Here's how the part is built. I have some questions about the finished solid (model axes, mm). A direction names the side the tool comes from. Coordinates: 2 decimals unless noted, no trailing zeros. Use a Markdown table: item, result.
Autodesk Inventor part; units mm, degrees
ref_plane "YZ Plane" through (0, 0, 0) normal (1, 0, 0) x (0, 1, 0)
ref_plane "XZ Plane" through (0, 0, 0) normal (0, 1, 0) x (-1, 0, 0)
ref_plane "XY Plane" through (0, 0, 0) normal (0, 0, 1) x (1, 0, 0)
sketch "Sketch1" plane through (0, 0, 0) normal (0, 1, 0) x (-1, 0, 0)
  arc A0 (5, 25) -> (25, 5) centre (25, 25) ccw
  circle A1 centre (25, 25) radius 20
  arc A2 (0, 10) -> (10, 0) centre (10, 10) ccw
  circle A3 centre (10, 10) radius 10
  line L0 (5.8856, 19.1144) -> (0, 19.1144)
  line L1 (0, 90) -> (0, 10)
  line L2 (19.1144, 5.8856) -> (19.1144, 0)
  line L3 (10, 0) -> (190, 0)
  line L4 (0, 19.1144) -> (19.1144, 19.1144)
  line L5 (19.1144, 19.1144) -> (19.1144, 0)
  line L6 (19.1144, 0) -> (0, 0)
  line L7 (0, 0) -> (0, 19.1144)
  arc A4 (45, 75) -> (5, 75) centre (25, 75) ccw
  circle A5 centre (25, 75) radius 20
  line L8 (25, 75) -> (25, 25)
  line L9 (25, 75) -> (35, 75)
  line L10 (35, 75) -> (35, 50)
  line L11 (35, 50) -> (25, 50)
  line L12 (25, 50) -> (25, 75)
  circle A6 centre (25, 75) radius 20
  line L13 (19.1144, 80.8856) -> (19.1144, 100)
  line L14 (0, 80.8856) -> (19.1144, 80.8856)
  line L15 (0, 100) -> (0, 80.8856)
  line L16 (19.1144, 100) -> (0, 100)
  circle A7 centre (10, 90) radius 10
  line L17 (19.1144, 0) -> (169.1144, 0) construction
  line L18 (-101.8121, -91.2055) -> (-91.2055, -101.8121)
  line L19 (0, 0) -> (-96.5088, -96.5088)
  line L20 (-96.5088, -96.5088) -> (-91.2055, -101.8121)
  line L21 (-91.2055, -101.8121) -> (-101.8121, -91.2055)
  line L22 (-91.2055, -101.8121) -> (10.6066, 0)
  line L23 (-101.8121, -91.2055) -> (0, 10.6066)
  line L24 (0, 19.1144) -> (-101.8121, -91.2055)
  line L25 (19.1144, 0) -> (-91.2055, -101.8121)
  point P0 (19.1144, 5.8856)
  point P1 (5.8856, 19.1144)
  point P2 (10, 100)
  point P3 (5.8856, 80.8856)
  point P4 (19.1144, 94.1144)
  point P5 (5.8856, 19.1144)
  point P6 (19.1144, 5.8856)
  dimension "d0" = 10
  dimension "d1" = 25
extrude "Extrusion1" add sketch "Sketch1" along normal blind 35 contours A0 A3 A2 | A3 L1 L0 | L2 L3 A3 | L7 L19 L18 L23 L1 | A2 L6 L7 | L1 L23 L24 | L3 L22 L18 L19 L6 | L25 L22 L3
sketch "Sketch3" plane through (0, 0, 0) normal (0, -1, 0) x (1, 0, 0)
  arc A0 (-19.1144, 5.8856) -> (-5.8856, 19.1144) centre (-25, 25) ccw
  circle A1 centre (-25, 25) radius 20
  line L0 (0, 0) -> (-19.1144, 0)
  line L1 (-19.1144, 0) -> (-19.1144, 19.1144)
  line L2 (-19.1144, 19.1144) -> (0, 19.1144)
  line L3 (0, 19.1144) -> (0, 0)
  line L4 (91.2055, -101.8121) -> (-19.1144, 0)
  line L5 (-5.8856, 19.1144) -> (0, 19.1144)
  line L6 (-19.1144, 0) -> (0, 19.1144)
  line L7 (-19.1144, 19.1144) -> (0, 0)
  point P0 (-5.8856, 19.1144)
  point P1 (-19.1144, 5.8856)
extrude "Extrusion4" cut sketch "Sketch3" against normal blind 20 contours A0 L7 L6 L1 | A0 L2 L6 L7 | L6 L7 L0 | L6 L3 L7
fillet "Fillet2" radius 10 1 edges at (0, 10, 0)
sketch "Sketch6" plane through (91.2055, 0, -101.8121) normal (-0.6782, 0, -0.7349) x (-0.7349, 0, 0.6782)
  line L0 (150.1206, 20) -> (150.1206, 35)
  line L1 (150.1206, 35) -> (136.6046, 35)
  line L2 (0, 35) -> (150.1206, 35)
  line L3 (143.4227, 0) -> (150.1206, 0)
  line L4 (0, 35) -> (150.1206, 35)
  line L5 (150.1206, 35) -> (150.1206, 0)
  line L6 (150.1206, 0) -> (0, 0)
  line L7 (0, 0) -> (0, 35)
  line L8 (0, 0) -> (150.1206, 0)
  line L9 (0, 0) -> (0, 10)
  line L10 (0, 0) -> (10, 0) construction
  line L11 (0, 10) -> (136.6046, 35)
  line L12 (0, 10) -> (-15.7766, 7.1127)
  line L13 (-15.7766, 7.1127) -> (-15.4206, 35)
  line L14 (0, 0) -> (0, 35)
  line L15 (-15.4206, 35) -> (0, 35)
  point P0 (136.0739, 0)
  dimension "d22" = 13.516
  dimension "d23" = 10
  dimension "d24" = 90
extrude "Extrusion5" cut sketch "Sketch6" against normal through all contours L11 L7 L2 | L7 L12 L13 L15
sketch "Sketch7" plane through (0, 20, 0) normal (0, -1, 0) x (1, 0, 0)
  line L0 (0, 0) -> (200, 0)
  line L1 (200, 0) -> (200, 100)
  line L2 (200, 100) -> (0, 100)
  line L3 (0, 100) -> (0, 0)
  line L4 (0, 0) -> (7, 0)
  line L5 (7, 0) -> (7, 7)
  line L6 (7, 7) -> (0, 7)
  line L7 (0, 7) -> (0, 0)
  line L8 (200, 100) -> (193, 100)
  line L9 (193, 100) -> (193, 93)
  line L10 (193, 93) -> (200, 93)
  line L11 (200, 93) -> (200, 100)
  line L12 (7, 7) -> (193, 7)
  line L13 (193, 7) -> (193, 93)
  line L14 (193, 93) -> (7, 93)
  line L15 (7, 93) -> (7, 7)
  line L16 (0, 0) -> (-200, 0)
  line L17 (-200, 0) -> (-200, 100)
  line L18 (-200, 100) -> (0, 100)
  line L19 (0, 0) -> (-7, 0)
  line L20 (-7, 0) -> (-7, 7)
  line L21 (-7, 7) -> (0, 7)
  line L22 (-200, 100) -> (-193, 100)
  line L23 (-193, 100) -> (-193, 93)
  line L24 (-193, 93) -> (-200, 93)
  line L25 (-200, 93) -> (-200, 100)
  line L26 (-7, 7) -> (-193, 7)
  line L27 (-193, 7) -> (-193, 93)
  line L28 (-193, 93) -> (-7, 93)
  line L29 (-7, 93) -> (-7, 7)
  dimension "d27" = 200
  dimension "d28" = 100
  dimension "d29" = 7
  dimension "d30" = 7
  dimension "d31" = 7
  dimension "d32" = 7
hole "Hole1" at (-7, 20, 7) direction (0, 1, 0) diameter 5 end through all
fillet "Fillet3" radius 5 1 edges at (96.5088, 9.945, -96.5088)
fillet "Fillet4" radius 5 4 edges at (90.3527, 9.0335, -101.025) (91.2055, 2.9156, -101.8121) (101.025, 8.9228, -90.3527) (101.8121, 2.8606, -91.2055)
sketch "Sketch8" plane through (0, 0, 0) normal (0, -1, 0) x (1, 0, 0)
  line L0 (98.4155, -94.6021) -> (94.6021, -98.4155)
  line L1 (98.4155, -94.6021) -> (103.9755, -89.0422)
  line L2 (0, 19.1144) -> (98.5544, -87.6756)
  line L3 (98.5544, -87.6756) -> (108.5515, -97.6726)
  ellipse E0 centre (94.88, -91.0666) end of major axis (91.3445, -87.531) minor radius 0.0367 (98.4155, -94.6021) -> (95.5415, -91.677) ccw
  line L4 (98.4155, -94.6021) -> (90.1473, -102.8703)
  line L5 (87.6756, -98.5544) -> (-19.1144, 0)
  line L6 (87.6756, -98.5544) -> (92.1576, -103.0365)
  circle A0 centre (90.9886, -90.9886) radius 7.8068
  circle A1 centre (90.9886, -90.9886) radius 20
  point P0 (0, 0)
  point P1 (98.0828, -94.2471)
  point P2 (96.5088, -96.5088)
  dimension "d42" = 40
extrude "Extrusion6" add sketch "Sketch8" against normal blind 5 contours L1 L3 L2 A1 L5 L6 L4 L0 | E0 A0 L2 L3 L1 | L0 L4 L6 L5 A0 | A0 | L5 A1 L2 A0
fillet "Fillet5" radius 5 1 edges at (105.1307, 5, -105.1307)
sketch "Sketch9" plane through (0, 0, 0) normal (0, -1, 0) x (1, 0, 0)
  arc A0 (72.1624, -84.2376) -> (84.2376, -72.1624) centre (90.9886, -90.9886) ccw
  circle A1 centre (90.9886, -90.9886) radius 4.25
  point P0 (0, 0)
  dimension "d46" = 8.5
extrude "Extrusion7" cut sketch "Sketch9" against normal through all
sketch "Sketch10" plane through (0, 0, 0) normal (0, -1, 0) x (1, 0, 0)
  circle A0 centre (90.9886, -90.9886) radius 4.25
  circle A1 centre (90.9886, -90.9886) radius 4.25
  circle A2 centre (90.9886, -90.9886) radius 2.5
  point P0 (0, 0)
  dimension "d49" = 5
extrude "Extrusion8" add sketch "Sketch10" against normal blind 5
properties part number "Noga"
Q1. If we mould it in two halves opening along Z, with no side actions, what happens to faces 4 (the face through (-4, 35, 7)), 5 (the face through (93, 5, -93)), 6 (the face through (-10.955, 27.395, 10.762))? For each: pulls with the +Z half, pulls with the -Z half, needs draft (parallel to the pull), parting line crosses it, or undercut.
Check values:
| item | result |
|---|---|
| face 4 | needs draft |
| face 5 | undercut |
| face 6 | pulls with the +Z half |
Q2. Which directions (+Z, -Z, +X, -X, +Y, -Y) give clear straight access to the entire face, cutting with the end or side of a thin tool? Please do faces 1 (the face through (97, 5, -97)), 2 (the face through (0, 10, 15)), 3 (the face through (35.091, 25.855, -34.872)).
Check values:
| item | result |
|---|---|
| face 1 | +Y |
| face 2 | +Z, -X, -Y |
| face 3 | -Z, +X, +Y |
Q3. Will these pins go through, and if not, where does the flat tip stop? P1, Ø4, axis at x = 91.5, z = -89.5, coming from the +Y side; P2, Ø4.5, axis at y = 8.5, z = 13, coming from the -X side; P3, Ø6, axis at y = 14, z = -74.5, coming from the +X side; P4, Ø8, axis at y = 28.5, z = -51.5, coming from the -X side.
Check values:
| item | result |
|---|---|
| P1 | y = 5 |
| P2 | x = 0 |
| P3 | x = 86.87 |
| P4 | through |
Q4. Please list where these lines run through material, in increasing order: L1, parallel to Y at x = 93, z = -102; L2, parallel to Y at x = 37, z = -22; L3, parallel to X at y = 20, z = -3. Write a range as from..to.
Check values:
| item | result |
|---|---|
| L1 | 0..5 |
| L2 | 0..24.76 |
| L3 | -15.86..20.41 |
